Geometry: final body of the model. Coordinates: model frame, mm. A direction names the side the tool comes from. Give positions to 0.01 mm unless a question says otherwise; leave off trailing zeros. Loops run counter-clockwise (first coordinate to the right, second up) from the corner with the lowest first, then second, coordinate; pieces in that order, holes last. Notation, with made-up numbers: (30, 41) -> (46, 41) arc R23 cw to (46, 54) -> close; hole circle Ø10 at (-12, 4.25). An arc over 180 degrees is marked (long way). Answer in a Markdown table with one row per item. Add a question column.
1) Access query for faces 4 (the flat face through (145, 10, 0)), 5 (the flat face through (146, 2, -11)). Directions: +Z, -Z, +X, -X, +Y, -Y. A direction counts if a zero-diameter tool reaches every point of the face in a straight line with its end or side. Return the directions, or none.
2) Line query: line 1 (Z direction, x = 113, y = 4.75); line 2 (Y direction, x = 116, z = -14); line 3 (X direction, y = 2.5, z = -1). Output: solid intervals per line, ascending. Write a range as from..to.
3) Draft query along X for faces 1 (the flat face through (5.5, 5.5, -1.8)), 2 (the flat face through (293.714, 1.805, -5.509)), 3 (the flat face through (145, 0, -10)). Return one class per face: +X half, -X half, draft (parallel to the pull), parting line (faces both ways), or undercut.
4) Section query A-A (x = 60). Return the cut outline in (y, z), plus the area to 3 significant figures.
5) Section query B-B (z = -9.75). Return the cut outline in (x, y).
6) Section query C-C (y = 4.75). Return the cut outline in (x, z).
7) First-contact query: P1, Ø10, axis at x = 257, z = -9, coming from the +Y side; P2, Ø5, axis at x = 206, y = 14, coming from the +Z side; P3, Ø5.5, axis at x = 134.5, y = 7, coming from the -Z side; P4, Ø1.5, axis at y = 3, z = -3, coming from the -X side. Flat tips, straight axial feed; report the tip coordinate or a pass-through.
```python
from build123d import *

# Parameters (mm, degrees)
BOSS_EXTRUDE1_DEPTH = 294
CUT_EXTRUDE1_DEPTH  = 296.357410606


with BuildPart() as part:
    # Sketch1 → Boss-Extrude1 (new body)
    with BuildSketch(Plane(origin=(0, 0, 0), x_dir=(0, 0, -1), z_dir=(1, 0, 0))):
        Polygon((0, 20), (0, 0), (20, 0), (20, 2), (2, 2), (2, 20), align=None)
    extrude(amount=BOSS_EXTRUDE1_DEPTH)

    # Sketch2 → Cut-Extrude1 (cut, through all)
    with BuildSketch(Plane(origin=(0, 0, 0), x_dir=(-1, 0, 0), z_dir=(0, 0, -1))):
        Polygon((0, 0), (-20, 20), (0, 20), align=None)
        Polygon((-294, 0), (-290.832311194, 20), (-294, 20), align=None)
    extrude(amount=CUT_EXTRUDE1_DEPTH, mode=Mode.SUBTRACT)


solid = part.part
```
Evaluation:
| question | item | result |
|---|---|---|
| 1 | face 4 | +Z, +X, -X, +Y, -Y |
| 1 | face 5 | -Z, +X, -X, +Y |
| 2 | line 1 | -2..0 |
| 2 | line 2 | 0..2 |
| 2 | line 3 | 2.5..293.6 |
| 3 | face 1 | -X half |
| 3 | face 2 | +X half |
| 3 | face 3 | draft |
| 4 | outline | (0, -20) -> (2, -20) -> (2, -2) -> (20, -2) -> (20, 0) -> (0, 0) -> close |
| 4 | area | 76.0 mm² |
| 5 | outline | (0, 0) -> (294, 0) -> (293.68, 2) -> (2, 2) -> close |
| 6 | outline | (4.75, -2) -> (293.25, -2) -> (293.25, 0) -> (4.75, 0) -> close |
| 7 | P1 | y = 2 |
| 7 | P2 | z = 0 |
| 7 | P3 | z = -2 |
| 7 | P4 | through |
